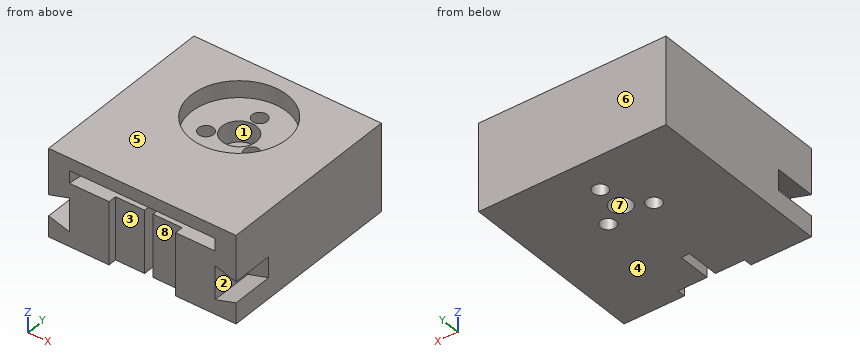
from build123d import *

# Parameters (mm, degrees)
SKETCH1_W           = 45
SKETCH1_H           = 45
BOSS_EXTRUDE1_DEPTH = 15
CUT_EXTRUDE1_DEPTH  = 66.383484153
CUT_EXTRUDE2_DEPTH  = 10.1
SKETCH4_W           = 45
SKETCH4_H           = 45
BOSS_EXTRUDE2_DEPTH = 3
SKETCH5_R           = 17.5
CUT_EXTRUDE3_DEPTH  = 3
SKETCH6_W           = 45
SKETCH6_H           = 45
BOSS_EXTRUDE3_DEPTH = 3
SKETCH7_R           = 2.6
CUT_EXTRUDE4_DEPTH  = 68.014923711
SKETCH8_R           = 1.8
CUT_EXTRUDE5_DEPTH  = 68.014923711
SKETCH9_R           = 11.5
CUT_EXTRUDE6_DEPTH  = 4
SKETCH10_R          = 4.1
CUT_EXTRUDE7_DEPTH  = 5


with BuildPart() as part:
    # Sketch1 → Boss-Extrude1 (new body)
    with BuildSketch(Plane.XY):
        with Locations((22.5, 22.5)):
            Rectangle(SKETCH1_W, SKETCH1_H)
    extrude(amount=BOSS_EXTRUDE1_DEPTH)

    # Sketch2 → Cut-Extrude1 (cut, through all)
    with BuildSketch(Plane.XY.offset(15)):
        Polygon((14.5, 0), (30.5, 0), (30.5, 2), (23.5, 2), (23.5, 10), (21.5, 10), (21.5, 2), (14.5, 2), align=None)
    extrude(amount=-CUT_EXTRUDE1_DEPTH, mode=Mode.SUBTRACT)

    # Sketch3 → Cut-Extrude2 (cut)
    with BuildSketch(Plane.XZ):
        Polygon((45, 10), (40, 11.5), (40, 3.5), (45, 5), align=None)
    cut_extrude2 = extrude(amount=-CUT_EXTRUDE2_DEPTH, mode=Mode.SUBTRACT)

    # Mirror1: Cut-Extrude2 across plane
    add(cut_extrude2.mirror(Plane(origin=(22.5, 0, 0), x_dir=(0, 0, 1), z_dir=(1, 0, 0))), mode=Mode.SUBTRACT)

    # Sketch4 → Boss-Extrude2 (add)
    with BuildSketch(Plane.XY.offset(15)):
        with Locations((22.5, 22.5)):
            Rectangle(SKETCH4_W, SKETCH4_H)
    extrude(amount=BOSS_EXTRUDE2_DEPTH)

    # Sketch5 → Cut-Extrude3 (cut)
    with BuildSketch(Plane.XY.offset(18)):
        with Locations((22.5, 0)):
            Circle(SKETCH5_R)
    extrude(amount=-CUT_EXTRUDE3_DEPTH, mode=Mode.SUBTRACT)

    # Sketch6 → Boss-Extrude3 (add)
    with BuildSketch(Plane.XY.offset(18)):
        with Locations((22.5, 22.5)):
            Rectangle(SKETCH6_W, SKETCH6_H)
    extrude(amount=BOSS_EXTRUDE3_DEPTH)

    # Sketch7 → Cut-Extrude4 (cut, through all)
    with BuildSketch(Plane.XY.offset(21)):
        with Locations((22.5, 30)):
            Circle(SKETCH7_R)
    extrude(amount=-CUT_EXTRUDE4_DEPTH, mode=Mode.SUBTRACT)

    # Sketch8 → Cut-Extrude5 (cut, through all)
    with BuildSketch(Plane.XY.offset(21)):
        with Locations((22.5, 36.35)):
            Circle(SKETCH8_R)
        with Locations((27.999261314, 26.825)):
            Circle(SKETCH8_R)
        with Locations((17.000738686, 26.825)):
            Circle(SKETCH8_R)
    extrude(amount=-CUT_EXTRUDE5_DEPTH, mode=Mode.SUBTRACT)

    # Sketch9 → Cut-Extrude6 (cut)
    with BuildSketch(Plane.XY.offset(21)):
        with Locations((22.5, 30)):
            Circle(SKETCH9_R)
    extrude(amount=-CUT_EXTRUDE6_DEPTH, mode=Mode.SUBTRACT)

    # Sketch10 → Cut-Extrude7 (cut)
    with BuildSketch(Plane.XY.offset(17)):
        with Locations((22.5, 30)):
            Circle(SKETCH10_R)
    extrude(amount=-CUT_EXTRUDE7_DEPTH, mode=Mode.SUBTRACT)


solid = part.part
Part model, mm, in its own coordinate system. Face numbers are marked on the shaded views. A direction names the side the tool comes from. Coordinates: 2 decimals unless noted, no trailing zeros. Order: outer loops, then holes, each group sorted by start corner. A loop starts at its lowest first (then second) coordinate and runs counter-clockwise, first axis right, second up. Notation, with made-up numbers: M 10.5,23 L 43.5,23 A15 ccw 43.5,41 Z; hole C 9.25,-34 d4. An arc over 180 degrees is marked long. Use a Markdown table: item, result.
(1) Flat gauge pins, fed straight in: pin 1 (1 mm diameter, centred on y = 1.5, z = 6, fed in from -X); pin 2 (6.5 mm diameter, centred on x = 24.5, y = 28.5, fed in from +Z); pin 3 (7 mm diameter, centred on x = 22.5, y = 30, fed in from +Z). Where does each tip first touch, or does it go through?
A:
| item | result |
|---|---|
| pin 1 | stops at x = 5 |
| pin 2 | stops at z = 17 |
| pin 3 | stops at z = 12 |
(2) Pull direction Y, two halves, no side cores. Call the marked faces 6, 7 and 8: released by +Y, released by -Y, zero draft, split by the parting line, or undercut.
A:
| item | result |
|---|---|
| face 6 | released by +Y |
| face 7 | undercut |
| face 8 | released by -Y |
(3) Probe L1, parallel to Y at x = 22.5, z = 8.75; L2, parallel to Y at x = 22.5, z = 13.75; L3, parallel to Z at x = 27, y = 9.5. List the from-to ranges inside material, lowest first.
A:
| item | result |
|---|---|
| L1 | y = 10 to 27.4, 32.6 to 34.55, 38.15 to 45 |
| L2 | y = 10 to 25.9, 34.1 to 34.55, 38.15 to 45 |
| L3 | z = 0 to 15, 18 to 21 |
(4) Tool access for the marked faces 1, 2, 3, 4 and 5: list every direction of +Z, -Z, +X, -X, +Y, -Y with a clear straight run to the whole face (end or side of a thin tool).
A:
| item | result |
|---|---|
| face 1 | +Z |
| face 2 | -Y |
| face 3 | -Z, -Y |
| face 4 | -Z, +X, -X, +Y, -Y |
| face 5 | +Z, +X, -X, +Y, -Y |
(5) Cut at C-C on y = 23.5. Write the cut outline in (x, z).
A:
| item | result |
|---|---|
| outline | M 0,0 L 45,0 L 45,21 L 31.99,21 L 31.99,17 L 13.01,17 L 13.01,21 L 0,21 Z |
(6) Cut at B-B on x = 22.5. Write the cut outline in (y, z), then the cut area to 3 significant figures.
A:
| item | result |
|---|---|
| outline | M 0,18 L 17.5,18 L 17.5,15 L 10,15 L 10,0 L 27.4,0 L 27.4,12 L 25.9,12 L 25.9,17 L 18.5,17 L 18.5,21 L 0,21 Z; M 32.6,0 L 34.55,0 L 34.55,17 L 34.1,17 L 34.1,12 L 32.6,12 Z; M 38.15,0 L 45,0 L 45,21 L 41.5,21 L 41.5,17 L 38.15,17 Z |
| area | 486 mm^2 |
(7) Cut at A-A on y = 30. Write the cut outline in (x, z).
A:
| item | result |
|---|---|
| outline | M 0,0 L 19.9,0 L 19.9,12 L 18.4,12 L 18.4,17 L 11,17 L 11,21 L 0,21 Z; M 25.1,0 L 45,0 L 45,21 L 34,21 L 34,17 L 26.6,17 L 26.6,12 L 25.1,12 Z |
(8) Cut at D-D on z = 4.25. Write the cut outline in (x, y) (3 decimals), then the cut area to 3 significant figures.
A:
| item | result |
|---|---|
| outline | M 0,0 L 2.5,0 L 2.5,10.1 L 5,10.1 L 5,0 L 14.5,0 L 14.5,2 L 21.5,2 L 21.5,10 L 23.5,10 L 23.5,2 L 30.5,2 L 30.5,0 L 40,0 L 40,10.1 L 42.5,10.1 L 42.5,0 L 45,0 L 45,45 L 0,45 Z; hole C 17.001,26.825 d3.6; hole C 22.5,30 d5.2; hole C 22.5,36.35 d3.6; hole C 27.999,26.825 d3.6 |
| area | 1,870 mm^2 |
